Model file for the job. Use its own axes, mm. Face numbers are marked on the shaded views. A direction names the side the tool comes from. Give positions to 0.01 mm unless a question says otherwise; leave off trailing zeros. Write each loop counter-clockwise with the first axis right and the second up, starting at its lowest first coordinate (ties: lowest second). Pieces come first, ordered by that corner, then holes. Notation, with made-up numbers: M 24.25,-25 L 49.25,-25 A21 cw 49.25,-7 Z; hole C 5.5,66 d7. An arc over 180 degrees is marked long. Answer as a JSON object with one key per item and string values. Group by question number.
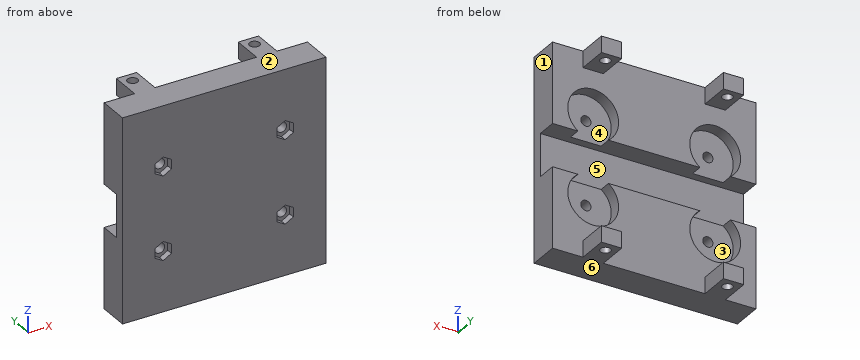
```python
from build123d import *

# Parameters (mm, degrees)
SKETCH1_W           = 1000
SKETCH1_H           = 1000
BOSS_EXTRUDE1_DEPTH = 300
SKETCH2_W           = 1000
SKETCH2_H           = 200
CUT_EXTRUDE1_DEPTH  = 100
MOVE_FACE1_BY       = 150
SCALE1_SCALE        = 0.1
SKETCH5_R           = 12.5
CUT_EXTRUDE4_DEPTH  = 6
SKETCH11_R          = 12.5
CUT_EXTRUDE5_DEPTH  = 6
SKETCH12_R          = 12.5
CUT_EXTRUDE6_DEPTH  = 6
SKETCH13_R          = 12.5
CUT_EXTRUDE7_DEPTH  = 6
CUT_EXTRUDE8_DEPTH  = 3
SKETCH15_R          = 2.5
CUT_EXTRUDE9_DEPTH  = 16
CUT_EXTRUDE10_DEPTH = 3
SKETCH17_R          = 2.5
CUT_EXTRUDE11_DEPTH = 10
CUT_EXTRUDE12_DEPTH = 3
SKETCH19_R          = 2.5
CUT_EXTRUDE13_DEPTH = 10
CUT_EXTRUDE14_DEPTH = 3
SKETCH21_R          = 2.5
CUT_EXTRUDE15_DEPTH = 10
SKETCH27_W          = 10
SKETCH27_H          = 8
BOSS_EXTRUDE3_DEPTH = 15
CUT_EXTRUDE21_REACH = 529.87
SKETCH28_R          = 2.5
SKETCH30_W          = 10
SKETCH30_H          = 8
BOSS_EXTRUDE4_DEPTH = 15
SKETCH31_R          = 2.5
CUT_EXTRUDE22_DEPTH = 8
SKETCH32_W          = 10
SKETCH32_H          = 8
BOSS_EXTRUDE5_DEPTH = 15
CUT_EXTRUDE23_START = -8
SKETCH33_R          = 2.5
CUT_EXTRUDE23_DEPTH = 8
SKETCH34_W          = 10
SKETCH34_H          = 8
BOSS_EXTRUDE6_DEPTH = 15
CUT_EXTRUDE24_START = -8
SKETCH35_R          = 2.5
CUT_EXTRUDE24_DEPTH = 8
SKETCH40_W          = 100
SKETCH40_H          = 10
CUT_EXTRUDE25_DEPTH = 0.5
SKETCH41_W          = 100
SKETCH41_H          = 10
CUT_EXTRUDE26_DEPTH = 0.5


with BuildPart() as part:
    # Sketch1 → Boss-Extrude1 (new body)
    with BuildSketch(Plane(origin=(0, 0, 0), x_dir=(1, 0, 0), z_dir=(0, 1, 0))):
        with Locations((-407.266206583, -460.379609426)):
            Rectangle(SKETCH1_W, SKETCH1_H)
    extrude(amount=BOSS_EXTRUDE1_DEPTH)

    # Sketch2 → Cut-Extrude1 (cut)
    with BuildSketch(Plane(origin=(0, 300, 0), x_dir=(1, 0, 0), z_dir=(0, 1, 0))):
        with Locations((-407.266206583, -460.379609426)):
            Rectangle(SKETCH2_W, SKETCH2_H)
    extrude(amount=-CUT_EXTRUDE1_DEPTH, mode=Mode.SUBTRACT)

    # Move Face1: a face moved inward by 150.0
    extrude(part.faces().sort_by_distance((-407.266206583, 0, 460.379609426))[0], amount=MOVE_FACE1_BY, dir=(0, 1, 0), mode=Mode.SUBTRACT)


with BuildPart() as part_1:
    # Scale1: scaled about (-407.266206583, 221.153846154, 460.379609426)
    add(part.part.scale(SCALE1_SCALE).moved(Location((-366.539585925, 199.038461539, 414.341648483))))

    # Sketch5 → Cut-Extrude4 (cut)
    with BuildSketch(Plane(origin=(0, 229.038461538, 0), x_dir=(1, 0, 0), z_dir=(0, 1, 0))):
        with Locations((-437.266206583, -439.879609426)):
            Circle(SKETCH5_R)
    extrude(amount=-CUT_EXTRUDE4_DEPTH, mode=Mode.SUBTRACT)

    # Sketch11 → Cut-Extrude5 (cut)
    with BuildSketch(Plane(origin=(0, 229.038461538, 0), x_dir=(1, 0, 0), z_dir=(0, 1, 0))):
        with Locations((-377.266206583, -439.879609426)):
            Circle(SKETCH11_R)
    extrude(amount=-CUT_EXTRUDE5_DEPTH, mode=Mode.SUBTRACT)

    # Sketch12 → Cut-Extrude6 (cut)
    with BuildSketch(Plane(origin=(0, 229.038461538, 0), x_dir=(1, 0, 0), z_dir=(0, 1, 0))):
        with Locations((-377.266206583, -480.879609426)):
            Circle(SKETCH12_R)
    extrude(amount=-CUT_EXTRUDE6_DEPTH, mode=Mode.SUBTRACT)

    # Sketch13 → Cut-Extrude7 (cut)
    with BuildSketch(Plane(origin=(0, 229.038461538, 0), x_dir=(1, 0, 0), z_dir=(0, 1, 0))):
        with Locations((-437.266206583, -480.879609426)):
            Circle(SKETCH13_R)
    extrude(amount=-CUT_EXTRUDE7_DEPTH, mode=Mode.SUBTRACT)

    # Sketch14 → Cut-Extrude8 (cut)
    with BuildSketch(Plane(origin=(0, 214.038461538, 0), x_dir=(-1, 0, 0), z_dir=(0, -1, 0))):
        Polygon((377.266206583, -444.527279093), (381.291206583, -442.20344426), (381.291206583, -437.555774593), (377.266206583, -435.231939759), (373.241206583, -437.555774593), (373.241206583, -442.20344426), align=None)
    extrude(amount=-CUT_EXTRUDE8_DEPTH, mode=Mode.SUBTRACT)

    # Sketch15 → Cut-Extrude9 (cut)
    with BuildSketch(Plane(origin=(0, 217.038461538, 0), x_dir=(-1, 0, 0), z_dir=(0, -1, 0))):
        with Locations(Location((377.266206583, -439.879609426, 0), (0, 0, 90))):
            Circle(SKETCH15_R)
    extrude(amount=-CUT_EXTRUDE9_DEPTH, mode=Mode.SUBTRACT)

    # Sketch16 → Cut-Extrude10 (cut)
    with BuildSketch(Plane(origin=(0, 214.038461538, 0), x_dir=(-1, 0, 0), z_dir=(0, -1, 0))):
        Polygon((437.266206583, -444.527279093), (441.291206583, -442.20344426), (441.291206583, -437.555774593), (437.266206583, -435.231939759), (433.241206583, -437.555774593), (433.241206583, -442.20344426), align=None)
    extrude(amount=-CUT_EXTRUDE10_DEPTH, mode=Mode.SUBTRACT)

    # Sketch17 → Cut-Extrude11 (cut)
    with BuildSketch(Plane(origin=(0, 217.038461538, 0), x_dir=(-1, 0, 0), z_dir=(0, -1, 0))):
        with Locations(Location((437.266206583, -439.879609426, 0), (0, 0, 90))):
            Circle(SKETCH17_R)
    extrude(amount=-CUT_EXTRUDE11_DEPTH, mode=Mode.SUBTRACT)

    # Sketch18 → Cut-Extrude12 (cut)
    with BuildSketch(Plane(origin=(0, 214.038461538, 0), x_dir=(-1, 0, 0), z_dir=(0, -1, 0))):
        Polygon((377.266206583, -485.527279093), (381.291206583, -483.20344426), (381.291206583, -478.555774593), (377.266206583, -476.231939759), (373.241206583, -478.555774593), (373.241206583, -483.20344426), align=None)
    extrude(amount=-CUT_EXTRUDE12_DEPTH, mode=Mode.SUBTRACT)

    # Sketch19 → Cut-Extrude13 (cut)
    with BuildSketch(Plane(origin=(0, 217.038461538, 0), x_dir=(-1, 0, 0), z_dir=(0, -1, 0))):
        with Locations(Location((377.266206583, -480.879609426, 0), (0, 0, 90))):
            Circle(SKETCH19_R)
    extrude(amount=-CUT_EXTRUDE13_DEPTH, mode=Mode.SUBTRACT)

    # Sketch20 → Cut-Extrude14 (cut)
    with BuildSketch(Plane(origin=(0, 214.038461538, 0), x_dir=(-1, 0, 0), z_dir=(0, -1, 0))):
        Polygon((437.266206583, -485.527279093), (441.291206583, -483.20344426), (441.291206583, -478.555774593), (437.266206583, -476.231939759), (433.241206583, -478.555774593), (433.241206583, -483.20344426), align=None)
    extrude(amount=-CUT_EXTRUDE14_DEPTH, mode=Mode.SUBTRACT)

    # Sketch21 → Cut-Extrude15 (cut)
    with BuildSketch(Plane(origin=(0, 217.038461538, 0), x_dir=(-1, 0, 0), z_dir=(0, -1, 0))):
        with Locations(Location((437.266206583, -480.879609426, 0), (0, 0, 90))):
            Circle(SKETCH21_R)
    extrude(amount=-CUT_EXTRUDE15_DEPTH, mode=Mode.SUBTRACT)

    # Sketch27 → Boss-Extrude3 (add)
    with BuildSketch(Plane(origin=(0, 229.038461538, 0), x_dir=(1, 0, 0), z_dir=(0, 1, 0))):
        with Locations((-437.266206583, -506.379609426)):
            Rectangle(SKETCH27_W, SKETCH27_H)
    extrude(amount=BOSS_EXTRUDE3_DEPTH)

    # Sketch28 → Cut-Extrude21 (cut, up to next)
    with BuildSketch(Plane.XY.offset(510.379609426), mode=Mode.PRIVATE) as cut_extrude21_sk1:
        with Locations((-437.266206583, 239.038461538)):
            Circle(SKETCH28_R)
    cut_extrude21_tool1 = extrude(cut_extrude21_sk1.sketch, amount=-CUT_EXTRUDE21_REACH, mode=Mode.PRIVATE) & part_1.part
    add(cut_extrude21_tool1.solids().sort_by_distance((-437.266207, 239.038462, 510.379609))[0], mode=Mode.SUBTRACT)

    # Sketch30 → Boss-Extrude4 (add)
    with BuildSketch(Plane(origin=(0, 229.038461538, 0), x_dir=(1, 0, 0), z_dir=(0, 1, 0))):
        with Locations((-377.266206583, -506.379609426)):
            Rectangle(SKETCH30_W, SKETCH30_H)
    extrude(amount=BOSS_EXTRUDE4_DEPTH)

    # Sketch31 → Cut-Extrude22 (cut)
    with BuildSketch(Plane.XY.offset(510.379609426)):
        with Locations((-377.266206583, 239.038461538)):
            Circle(SKETCH31_R)
    extrude(amount=-CUT_EXTRUDE22_DEPTH, mode=Mode.SUBTRACT)

    # Sketch32 → Boss-Extrude5 (add)
    with BuildSketch(Plane(origin=(0, 229.038461538, 0), x_dir=(1, 0, 0), z_dir=(0, 1, 0))):
        with Locations((-437.266206583, -414.379609426)):
            Rectangle(SKETCH32_W, SKETCH32_H)
    extrude(amount=BOSS_EXTRUDE5_DEPTH)

    # Sketch33 → Cut-Extrude23 (cut)
    with BuildSketch(Plane(origin=(0, 0, 410.379609426), x_dir=(-1, 0, 0), z_dir=(0, 0, -1)).offset(CUT_EXTRUDE23_START)):
        with Locations(Location((437.266206583, 239.038461538, 0), (0, 0, 180))):
            Circle(SKETCH33_R)
    extrude(amount=CUT_EXTRUDE23_DEPTH, mode=Mode.SUBTRACT)

    # Sketch34 → Boss-Extrude6 (add)
    with BuildSketch(Plane(origin=(0, 229.038461538, 0), x_dir=(1, 0, 0), z_dir=(0, 1, 0))):
        with Locations((-377.266206583, -414.379609426)):
            Rectangle(SKETCH34_W, SKETCH34_H)
    extrude(amount=BOSS_EXTRUDE6_DEPTH)

    # Sketch35 → Cut-Extrude24 (cut)
    with BuildSketch(Plane(origin=(0, 0, 410.379609426), x_dir=(-1, 0, 0), z_dir=(0, 0, -1)).offset(CUT_EXTRUDE24_START)):
        with Locations(Location((377.266206583, 239.038461538, 0), (0, 0, 180))):
            Circle(SKETCH35_R)
    extrude(amount=CUT_EXTRUDE24_DEPTH, mode=Mode.SUBTRACT)

    # Sketch40 → Cut-Extrude25 (cut)
    with BuildSketch(Plane(origin=(0, 0, 470.379609426), x_dir=(-1, 0, 0), z_dir=(0, 0, -1))):
        with Locations((407.266206583, 224.038461538)):
            Rectangle(SKETCH40_W, SKETCH40_H)
    extrude(amount=-CUT_EXTRUDE25_DEPTH, mode=Mode.SUBTRACT)

    # Sketch41 → Cut-Extrude26 (cut)
    with BuildSketch(Plane.XY.offset(450.379609426)):
        with Locations((-407.266206583, 224.038461538)):
            Rectangle(SKETCH41_W, SKETCH41_H)
    extrude(amount=-CUT_EXTRUDE26_DEPTH, mode=Mode.SUBTRACT)


solid = part_1.part
```
Q1. Drop flat-ended pins along their axis: P1, Ø4, axis at x = -377.27, z = 439.88, coming from the -Y side; P2, Ø2, axis at x = -399, z = 421, coming from the +Y side; P3, Ø9, axis at y = 236.5, z = 412.5, coming from the +X side; P4, Ø4, axis at y = 238, z = 414.5, coming from the -X side. Give the stop position or say it passes through.
Q2. Slice it at D-D, the plane z = 446. Write the cut outline in (x, y).
Q3. Slice it at B-B, the plane x = -415.5. Write the cut outline in (y, z), then the cut area to 3 significant figures.
Q4. Two-plate mould, pull along Z, no slides. Class the marked faces 1, 2 and 3: +Z half, -Z half, draft (parallel to the pull), parting line (faces both ways), or undercut.
Q5. Wall check: L1, parallel to Z at x = -397.5, y = 227.5; L2, parallel to Z at x = -435.5, y = 231; L3, parallel to Y at x = -392, z = 419. Give the ranges that are in metal, low to high.
Q6. Slice it at A-A, the plane y = 233. Write the cut outline in (x, z), then the cut area to 3 significant figures.
Q7. 3-axis set-ups, long thin cutter, end or side, ignore diameter. For the marked faces 4, 5 and 6: which of +Z, -Z, +X, -X, +Y, -Y reach the whole face in a straight line?
Q8. Slice it at C-C, the plane z = 425. Write the cut outline in (x, y).
Solved:
{
 "1": {"P1": "passes through", "P2": "stops at y = 229.04", "P3": "stops at x = -372.27", "P4": "stops at x = -442.27"},
 "2": {"outline": "M -457.27,214.04 L -357.27,214.04 L -357.27,229.04 L -366.37,229.04 L -366.37,223.04 L -388.17,223.04 L -388.17,229.04 L -426.37,229.04 L -426.37,223.04 L -448.17,223.04 L -448.17,229.04 L -457.27,229.04 Z"},
 "3": {"outline": "M 214.04,410.38 L 229.04,410.38 L 229.04,449.88 L 219.04,449.88 L 219.04,470.88 L 229.04,470.88 L 229.04,510.38 L 214.04,510.38 Z", "area": "1,290 mm²"},
 "4": {"face 1": "draft", "face 2": "+Z half", "face 3": "undercut"},
 "5": {"L1": "z = 410.38 to 449.88, 470.88 to 510.38", "L2": "z = 410.38 to 418.38, 502.38 to 510.38", "L3": "y = 214.04 to 229.04"},
 "6": {"outline": "M -442.27,410.38 L -432.27,410.38 L -432.27,418.38 L -442.27,418.38 Z; M -442.27,502.38 L -432.27,502.38 L -432.27,510.38 L -442.27,510.38 Z; M -382.27,410.38 L -372.27,410.38 L -372.27,418.38 L -382.27,418.38 Z; M -382.27,502.38 L -372.27,502.38 L -372.27,510.38 L -382.27,510.38 Z", "area": "320 mm²"},
 "7": {"face 4": "+Y", "face 5": "+X, -X, +Y", "face 6": "-Z, +X, -X, +Y, -Y"},
 "8": {"outline": "M -457.27,214.04 L -357.27,214.04 L -357.27,229.04 L -457.27,229.04 Z"}
}
